For this review, take the finished solid that the model builds, in its own axes (mm). A direction names the side the tool comes from. Coordinates: 2 decimals unless noted, no trailing zeros. Write each loop counter-clockwise with the first axis right and the second up, starting at its lowest first coordinate (ties: lowest second). Pieces come first, ordered by that corner, then holes.
```python
from build123d import *

# Parameters (mm, degrees)
BOSS_EXTRUDE1_DEPTH = 12.7
CUT_EXTRUDE1_DEPTH  = 38.486519244
FILLET4_R           = 1.524
FILLET5_R           = 3.81
SKETCH3_R           = 1.27
CUT_EXTRUDE2_DEPTH  = 68.465574925
SKETCH4_W           = 5.08
SKETCH4_H           = 9.652
CUT_EXTRUDE3_DEPTH  = 38.486519401
FILLET6_R           = 2.54


with BuildPart() as part:
    # Sketch1 → Boss-Extrude1 (new body)
    with BuildSketch(Plane(origin=(0, 0, 0), x_dir=(1, 0, 0), z_dir=(0, 1, 0))):
        Polygon((5.842, 32.385), (-13.97, 32.385), (-13.97, -32.385), (5.842, -32.385), (5.842, -24.765), (-1.27, -24.765), (-1.27, -20.193), (-5.08, -20.193), (-5.08, -12.573), (-1.27, -12.573), (5.842, -12.573), (13.97, -12.573), (13.97, 12.573), (5.842, 12.573), (-1.27, 12.573), (-5.08, 12.573), (-5.08, 20.193), (-1.27, 20.193), (-1.27, 24.765), (5.842, 24.765), align=None)
    extrude(amount=BOSS_EXTRUDE1_DEPTH)

    # Sketch2 → Cut-Extrude1 (cut, through all)
    with BuildSketch(Plane(origin=(0, 12.7, 0), x_dir=(1, 0, 0), z_dir=(0, 1, 0))):
        Polygon((-1.27, 24.765), (5.842, 26.019037487), (5.842, 24.765), align=None)
        Polygon((-1.27, -24.765), (5.842, -26.019037487), (5.842, -24.765), align=None)
        Polygon((-1.27, 12.573), (13.97, 8.489454307), (13.97, 12.573), align=None)
        Polygon((-1.27, -12.573), (13.97, -8.489454307), (13.97, -12.573), align=None)
    extrude(amount=-CUT_EXTRUDE1_DEPTH, mode=Mode.SUBTRACT)

    # Fillet4
    fillet4_edges = [part.edges().sort_by_distance(p)[0] for p in [
        (-5.08, 6.35, 20.193),
        (-1.27, 6.35, 20.193),
        (-1.27, 6.35, -20.193),
        (-5.08, 6.35, -20.193),
        (-5.08, 6.35, -12.573),
        (-5.08, 6.35, 12.573),
    ]]
    fillet(fillet4_edges, radius=FILLET4_R)

    # Fillet5
    # the kernel refuses this fillet: 3.81 mm, written as the material it takes off along each edge
    with BuildSketch(Plane(origin=(-13.97, -9.525, 32.385), x_dir=(0, 0, -1), z_dir=(0, 1, 0)), Plane(origin=(-13.97, -9.525, -32.385), x_dir=(1, 0, 0), z_dir=(0, 1, 0)), Plane(origin=(5.842, -9.525, -32.385), x_dir=(0, 0, 1), z_dir=(0, 1, 0)), Plane(origin=(5.842, -9.525, 32.385), x_dir=(-1, 0, 0), z_dir=(0, 1, 0))) as fillet5_piece_1:
        with BuildLine():
            CenterArc((FILLET5_R, -FILLET5_R), FILLET5_R, 90, 90)
            Line((0, -FILLET5_R), (0, 0))
            Line((0, 0), (FILLET5_R, 0))
        make_face()
    extrude(amount=31.75, mode=Mode.SUBTRACT)
    with BuildSketch(Plane(origin=(5.842, 20.692423987, -26.019037487), x_dir=(-0.9848077530122095, 0, 0.17364817766692292), z_dir=(0, -1, 0)), Plane(origin=(5.842, 20.692423987, 26.019037487), x_dir=(0, 0, 1), z_dir=(0, -1, 0))) as fillet5_piece_2:
        with BuildLine():
            CenterArc((FILLET5_R * 0.839099631177, FILLET5_R), FILLET5_R, 190, 80)
            Line((-FILLET5_R * 0.145708121835, FILLET5_R * 0.826351822333), (0, 0))
            Line((0, 0), (FILLET5_R * 0.839099631177, 0))
        make_face()
    extrude(amount=28.684847974, mode=Mode.SUBTRACT)

    # Sketch3 → Cut-Extrude2 (cut, through all)
    with BuildSketch(Plane.XY.offset(32.385)):
        with Locations(Location((-9.391956596, 6.35, 0), (0, 0, 127.211471896))):
            Circle(SKETCH3_R)
    extrude(amount=-CUT_EXTRUDE2_DEPTH, mode=Mode.SUBTRACT)

    # Sketch4 → Cut-Extrude3 (cut, through all)
    with BuildSketch(Plane(origin=(0, 12.7, 0), x_dir=(1, 0, 0), z_dir=(0, 1, 0))):
        with Locations((9.652, 1.397)):
            Rectangle(SKETCH4_W, SKETCH4_H)
    extrude(amount=-CUT_EXTRUDE3_DEPTH, mode=Mode.SUBTRACT)

    # Fillet6
    fillet6_edges = [part.edges().sort_by_distance(p)[0] for p in [
        (-1.27, 6.35, 12.573),
        (13.97, 6.35, 8.489454307),
        (-1.27, 6.35, -12.573),
        (13.97, 6.35, -8.489454307),
    ]]
    fillet(fillet6_edges, radius=FILLET6_R)


solid = part.part
```
1) Consider section A-A (z = -5.5). Give the boundary of the cut face in (x, y), then the cut area to 3 significant figures.
2) Consider section D-D (z = 22.5). Give the boundary of the cut face in (x, y).
3) Consider section C-C (y = 6.35). Count the separate pieces of the cut face and the enclosed holes in it, then the cut area to 3 significant figures.
4) Consider section B-B (x = 10). Give the boundary of the cut face in (y, z).
5) Clearance check with flat-ended pins moving along their axes: P1, Ø5, axis at y = 4, z = 15.5, coming from the +X side; P2, Ø2.5, axis at x = 10.5, y = 3.5, coming from the -Z side; P3, Ø2, axis at x = -9.39, y = 6.35, coming from the +Z side; P4, Ø1.5, axis at x = 8.5, y = 5.5, coming from the +Z side. State where each tip first meets the part, or that it passes through.
6) For L1, parallel to X at y = 6.35, z = 2; L2, parallel to X at y = 2.5, z = -3; L3, parallel to Y at x = -9.25, z = 18.5, list the stretches that pass through material, from the lowest coordinate up.
7) Tool access review of faces 1 (the face through (7.112, 6, -1)), 2 (the face through (-3, 12.7, 0)), 3 (the face through (-1.728, 6.439, 20.628)): name each direction out of +Z, -Z, +X, -X, +Y, -Y from which nothing blocks a thin tool from reaching the whole face with its end or side.
8) The part is to be moulded in two halves that separate along Z. For faces 4 (the face through (5.479, 6.439, 10.765)), 5 (the face through (4.58, 6.26, 31.41)), 6 (the face through (-9.71, 7.58, 0.45)), say which applies: pulls with the +Z half, pulls with the -Z half, needs draft (parallel to the pull), parting line crosses it, or undercut.
Results:
1. outline: (-13.97, 0) - (7.11, 0) - (7.11, 12.7) - (-13.97, 12.7) - close; (12.19, 0) - (13.97, 0) - (13.97, 12.7) - (12.19, 12.7) - close; hole circle Ø2.54 at (-9.39, 6.35)
1. area: 285 mm2
2. outline: (-13.97, 0) - (-1.27, 0) - (-1.27, 12.7) - (-13.97, 12.7) - close; hole circle Ø2.54 at (-9.39, 6.35)
3. separate pieces: 2
3. enclosed holes: 1
3. area: 954 mm2
4. outline: (0, -9.55) - (12.7, -9.55) - (12.7, -6.22) - (0, -6.22) - close; (0, 3.43) - (12.7, 3.43) - (12.7, 9.55) - (0, 9.55) - close
5. P1: stops at x = -4.61
5. P2: stops at z = -9.75
5. P3: passes through
5. P4: stops at z = 10.16
6. L1: x = -13.97 to -10.66, -8.12 to 7.11, 12.19 to 13.97
6. L2: x = -13.97 to 7.11, 12.19 to 13.97
6. L3: y = 0 to 5.09, 7.61 to 12.7
7. face 1: +Y, -Y
7. face 2: +Z, -Z, +X, -X, +Y
7. face 3: +X, +Y, -Y
8. face 4: undercut
8. face 5: pulls with the +Z half
8. face 6: needs draft
